```python
from build123d import *

# Parameters (mm, degrees)
SKETCH1_W           = 60
SKETCH1_H           = 160
BOSS_EXTRUDE1_DEPTH = 3.175
SKETCH4_W           = 3.175
SKETCH4_H           = 9
SKETCH4_H_2         = 20
SKETCH4_W_2         = 15
SKETCH4_H_3         = 3.175
CUT_EXTRUDE2_DEPTH  = 3.175
SKETCH5_R           = 3.5
SKETCH5_R_2         = 1.7
CUT_EXTRUDE3_DEPTH  = 3.175
SKETCH6_R           = 5
SKETCH6_R_2         = 4.25
SKETCH6_W           = 9
SKETCH6_H           = 16
CUT_EXTRUDE4_DEPTH  = 3.175


with BuildPart() as part:
    # Sketch1 → Boss-Extrude1 (new body)
    with BuildSketch(Plane.XY):
        with Locations((-26.825, 54.431521206)):
            Rectangle(SKETCH1_W, SKETCH1_H)
    extrude(amount=-BOSS_EXTRUDE1_DEPTH)

    # Sketch4 → Cut-Extrude2 (cut)
    with BuildSketch(Plane.XY):
        with Locations((1.5875, -21.068478794)):
            Rectangle(SKETCH4_W, SKETCH4_H)
        with Locations((1.5875, 13.931521206)):
            Rectangle(SKETCH4_W, SKETCH4_H_2)
        with Locations((1.5875, 54.431521206)):
            Rectangle(SKETCH4_W, SKETCH4_H_2)
        with Locations((1.5875, 94.931521206)):
            Rectangle(SKETCH4_W, SKETCH4_H_2)
        with Locations((1.5875, 129.931521206)):
            Rectangle(SKETCH4_W, SKETCH4_H)
        with Locations((-39.475, -23.980978794)):
            Rectangle(SKETCH4_W_2, SKETCH4_H_3)
        with Locations((-55.2375, 13.931521206)):
            Rectangle(SKETCH4_W, SKETCH4_H_2)
        with Locations((-55.2375, 54.431521206)):
            Rectangle(SKETCH4_W, SKETCH4_H_2)
        with Locations((-55.2375, 94.931521206)):
            Rectangle(SKETCH4_W, SKETCH4_H_2)
        with Locations((-55.2375, 129.931521206)):
            Rectangle(SKETCH4_W, SKETCH4_H)
        with Locations((-55.2375, -21.068478794)):
            Rectangle(SKETCH4_W, SKETCH4_H)
        with Locations((-14.175, -23.980978794)):
            Rectangle(SKETCH4_W_2, SKETCH4_H_3)
        with Locations((-14.175, 132.844021206)):
            Rectangle(SKETCH4_W_2, SKETCH4_H_3)
        with Locations((-39.475, 132.844021206)):
            Rectangle(SKETCH4_W_2, SKETCH4_H_3)
    extrude(amount=-CUT_EXTRUDE2_DEPTH, mode=Mode.SUBTRACT)

    # Sketch5 → Cut-Extrude3 (cut)
    with BuildSketch(Plane.XY):
        with Locations((-12.75, -9.643478794)):
            Circle(SKETCH5_R)
        with Locations((-12.75, -18.143478794)):
            Circle(SKETCH5_R_2)
        with Locations(Location((-12.75, -1.143478794, 0), (0, 0, 180))):
            Circle(SKETCH5_R_2)
        with Locations(Location((-12.75, 127.006521206, 0), (0, 0, 180))):
            Circle(SKETCH5_R_2)
        with Locations(Location((-12.75, 118.506521206, 0), (0, 0, 180))):
            Circle(SKETCH5_R)
        with Locations((-12.75, 110.006521206)):
            Circle(SKETCH5_R_2)
    extrude(amount=-CUT_EXTRUDE3_DEPTH, mode=Mode.SUBTRACT)

    # Sketch6 → Cut-Extrude4 (cut)
    with BuildSketch(Plane.XY):
        with Locations((-33.75, 52.606521206)):
            Circle(SKETCH6_R)
        with Locations((-13.25, 70.106521206)):
            Circle(SKETCH6_R_2)
        with Locations((-33.75, 70.106521206)):
            Circle(SKETCH6_R)
        with Locations((-13.25, 52.606521206)):
            Rectangle(SKETCH6_W, SKETCH6_H)
    extrude(amount=-CUT_EXTRUDE4_DEPTH, mode=Mode.SUBTRACT)


solid = part.part
```
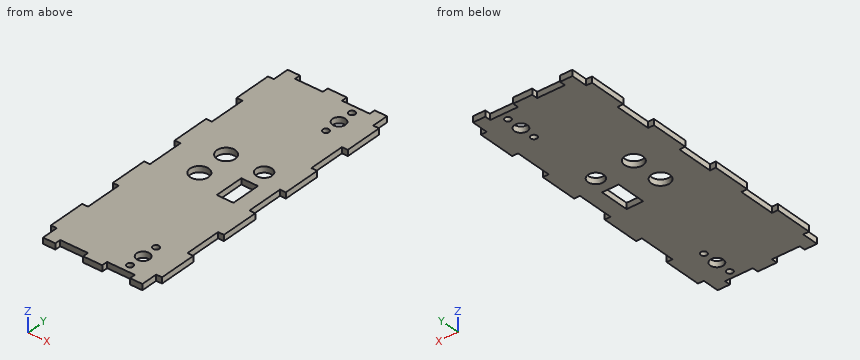
The listing builds one solid part. Answer for the finished solid, in the listing's coordinates (mm). Give positions to 0.01 mm unless a question says otherwise; leave off trailing zeros. Order: outer loops, then holes, each group sorted by start corner. A loop starts at its lowest first (then second) coordinate and runs counter-clockwise, first axis right, second up. Notation, with made-up numbers: (46.5, 8.25) -> (86.5, 8.25) arc R28 ccw to (86.5, 44.25) -> close; hole circle Ø10 at (78.25, 12.5). An arc over 180 degrees is marked (long way). Write each question's results on one line, items separated by ' | '.
Q1. The part is cut by section C-C, the plane x = -45.5. Give the vertices of the cut face in (y, z) (3 decimals).
Checked values:
outline: (-22.393, -3.175) -> (131.257, -3.175) -> (131.257, 0) -> (-22.393, 0) -> close
Q2. The part is cut by section B-B, the plane y = -8. Give the vertices of the cut face in (x, z) (3 decimals), and give its area (3 significant figures).
Checked values:
outline: (-56.825, -3.175) -> (-15.84, -3.175) -> (-15.84, 0) -> (-56.825, 0) -> close; (-9.66, -3.175) -> (3.175, -3.175) -> (3.175, 0) -> (-9.66, 0) -> close | area: 171 mm^2
Q3. Each of these flat-tipped pins is pushed along its axis until it touches: P1, Ø1.6, axis at x = 1, z = -2.5, coming from the -Y side; P2, Ø1.5, axis at y = 6, z = -2, coming from the +X side; P3, Ø8, axis at x = -33.75, y = 70.11, coming from the -Z side; P4, Ø1.6, axis at y = 133.5, z = -2, coming from the -X side. Where does it stop, or does it pass through?
Checked values:
P1: stops at y = -16.57 | P2: stops at x = 0 | P3: passes through | P4: stops at x = -53.65
Q4. The part is cut by section D-D, the plane z = -1.8. State how many separate pieces and enclosed holes the cut face has, and give its area (3 significant figures).
Checked values:
separate pieces: 1 | enclosed holes: 10 | area: 8,440 mm^2
Q5. The part is cut by section A-A, the plane x = -33.75. Give the vertices of the cut face in (y, z) (3 decimals), and give its area (3 significant figures).
Checked values:
outline: (-22.393, -3.175) -> (47.607, -3.175) -> (47.607, 0) -> (-22.393, 0) -> close; (57.607, -3.175) -> (65.107, -3.175) -> (65.107, 0) -> (57.607, 0) -> close; (75.107, -3.175) -> (131.257, -3.175) -> (131.257, 0) -> (75.107, 0) -> close | area: 424 mm^2
Q6. Straight lines are drawn through the part: probe 1 along Y at (x, z) = (-33.75, -1.4); probe 2 along Y at (x, z) = (-54, -0.25); probe 3 along Y at (x, z) = (-31.5, -1.3). For each, find the intervals that lie inside material, in ascending order. Write a range as from..to.
Checked values:
probe 1: y = -22.39..47.61, 57.61..65.11, 75.11..131.26 | probe 2: y = -16.57..3.93, 23.93..44.43, 64.43..84.93, 104.93..125.43 | probe 3: y = -25.57..48.14, 57.07..65.64, 74.57..134.43
